Model file for the job. Use its own axes, mm. Face numbers are marked on the shaded views. A direction names the side the tool comes from. Give positions to 0.01 mm unless a question says otherwise; leave off trailing zeros. Order: outer loops, then holes, each group sorted by start corner. A loop starts at its lowest first (then second) coordinate and runs counter-clockwise, first axis right, second up. Notation, with made-up numbers: (66, 19.5) - (123, 19.5) arc R10 ccw to (123, 31.5) - close; hole circle Ø9 at (56.25, 34.5). An arc over 180 degrees is marked (long way). Use CSV: the item, a comma, the result in double quotes. Start each with the question number.
(1) Band-saw the part on C-C, the plane y = 5.5. Give the cut face in (x, z).
(2) Drop flat-ended pins along their axis: pin 1 Ø6 at (x, z) = (-13.5, 13.5) entering from +Y; pin 2 Ø1.7 at (y, z) = (-0.5, 119) entering from +X; pin 3 Ø6 at (x, z) = (58.5, 65) entering from -Y. Give the stop position or say it passes through.
(3) Band-saw the part on B-B, the plane x = -6.5. Give the cut face in (y, z).
(4) Tool access for the marked faces 5, 6 and 7: list every direction of +Z, -Z, +X, -X, +Y, -Y with a clear straight run to the whole face (end or side of a thin tool).
(5) Band-saw the part on A-A, the plane z = 12. Give the cut face in (x, y).
(6) Band-saw the part on D-D, the plane x = -44. Give the cut face in (y, z).
(7) Pull direction Z, two halves, no side cores. Call the marked faces 1, 2, 3 and 4: +Z half, -Z half, draft (parallel to the pull), parting line (faces both ways), or undercut.
(8) Probe L1, parallel to Z at x = 18.5, y = 8; L2, parallel to X at y = -4.5, z = 7.5; L3, parallel to Y at x = 47, z = 76.5. List the from-to ranges inside material, lowest first.
from build123d import *

# Parameters (mm, degrees)
F0_W         = 153.0012339354
F0_H         = 58.951575309
F1_DEPTH     = 20.32
F2_R         = 29.4340917525
F3_R         = 29.3662882484
F3_R_2       = 9.1215869303
F4_DEPTH     = 84.582
F5_DEPTH     = 84.583
F6_R         = 12.0800155098
F7_DEPTH     = 84.583
F9_W         = 152.801066637
F9_H         = 59.5563165843
F10_DEPTH    = 19.812
F11_R        = 10.3122867818
F12_DEPTH    = 124.461
F13_T1_DEPTH = 173.1145612107
F14_R        = 26.9812507731
F15_R        = 9.5592417263
F16_DEPTH    = 124.461


# Not quite as in the source:
# - a fillet or chamfer that OpenCascade refuses, or shapes differently, is made with other operations: its cross-section is extruded or revolved along the edge and cut away or added


with BuildPart() as f1:
    # F0 (on Top) → F1 (new body)
    with BuildSketch(Plane.XY):
        Rectangle(F0_W, F0_H)
    extrude(amount=F1_DEPTH)

    # F2
    f2_edges = [f1.edges().sort_by_distance(p)[0] for p in [
        (-76.500617, -29.475788, 10.16),
        (-76.500617, 29.475788, 10.16),
        (76.500617, -29.475788, 10.16),
        (76.500617, 29.475788, 10.16),
    ]]
    fillet(f2_edges, radius=F2_R)

    # F3 (on face) → F4 (join)
    with BuildSketch(Plane.XY.offset(20.32)):
        with Locations((47.0665252152, 0.0416959021)):
            Circle(F3_R)
        with Locations((47.0665252152, 0.0416959021)):
            Circle(F3_R_2, mode=Mode.SUBTRACT)
    extrude(amount=F4_DEPTH)

    # F5 (cut, through all): a face of the model
    f5_faces = [f1.faces().sort_by_distance(p)[0] for p in [
        (47.0665252152, 0.0416959021, 20.32),
    ]]
    extrude(f5_faces, amount=F5_DEPTH, mode=Mode.SUBTRACT)

    # F6 (on face) → F7 (cut, through all)
    with BuildSketch(Plane.XY.offset(20.32)):
        with Locations((-47.0665252152, 0.0416959021)):
            Circle(F6_R)
    extrude(amount=F7_DEPTH, mode=Mode.SUBTRACT)

    # F9 (on offset) → F10 (join)
    with BuildSketch(Plane.XY.offset(104.648)):
        Rectangle(F9_W, F9_H)
    extrude(amount=F10_DEPTH)

    # F11 (on face) → F12 (cut, through all)
    with BuildSketch(Plane(origin=(0, 0, 0), x_dir=(1, 0, 0), z_dir=(0, 0, -1))):
        with Locations((-47.0665252152, 0.0416959021)):
            Circle(F11_R)
    extrude(amount=-F12_DEPTH, mode=Mode.SUBTRACT)

    # F13: fillet of radius 30.6605122421 on 2 edges, made by hand

    # F13_s2 → F13_t1 (cut)
    with BuildSketch(Plane.XY.offset(27.9967193947)):
        with BuildLine():
            ThreePointArc((-45.7400210764, -29.7781582922), (-67.4202771975, -20.7979021711), (-76.4005333185, 0.88235395))
            Line((-76.4005333185, 0.88235395), (-76.4005333185, -29.7781582922))
            Line((-76.4005333185, -29.7781582922), (-45.7400210764, -29.7781582922))
        make_face()
        with BuildLine():
            ThreePointArc((-45.7400210764, 29.7781582922), (-67.4202771975, 20.7979021711), (-76.4005333185, -0.88235395))
            Line((-76.4005333185, -0.88235395), (-76.4005333185, 29.7781582922))
            Line((-76.4005333185, 29.7781582922), (-45.7400210764, 29.7781582922))
        make_face()
    extrude(amount=F13_T1_DEPTH, mode=Mode.SUBTRACT)

    # F14
    f14_edges = [f1.edges().sort_by_distance(p)[0] for p in [
        (76.400533, -29.778158, 114.554),
        (76.400533, 29.778158, 114.554),
    ]]
    fillet(f14_edges, radius=F14_R)

    # F15 (on face) → F16 (cut, through all)
    with BuildSketch(Plane(origin=(0, 0, 0), x_dir=(1, 0, 0), z_dir=(0, 0, -1))):
        with Locations((56.2476292253, 0)):
            Circle(F15_R)
    extrude(amount=-F16_DEPTH, mode=Mode.SUBTRACT)


solid = f1.part
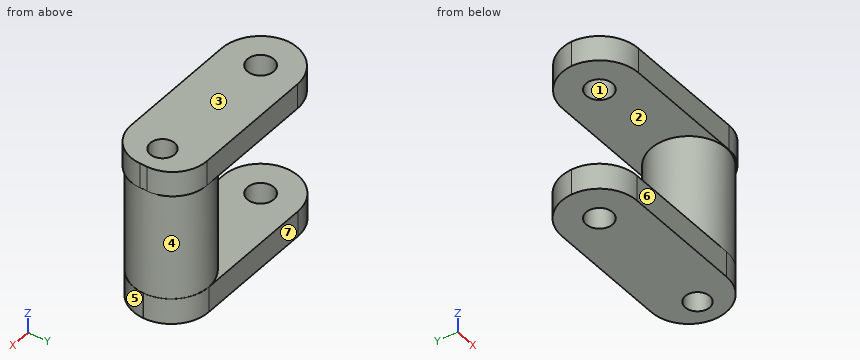
Answer block:
1,outline,"(-75.99, 0) - (-55.76, 0) - (-55.76, 20.32) - (-75.99, 20.32) - close; (-75.73, 104.65) - (-55.76, 104.65) - (-55.76, 124.46) - (-75.73, 124.46) - close; (-38.37, 0) - (48.43, 0) - (48.43, 20.32) - (39.76, 20.32) - (39.76, 104.65) - (48.43, 104.65) - (48.43, 124.46) - (-38.37, 124.46) - (-38.37, 104.65) - (18.21, 104.65) - (18.21, 20.32) - (-38.37, 20.32) - close; (64.07, 0) - (75.99, 0) - (75.99, 20.32) - (75.92, 20.32) - (75.92, 104.65) - (76.26, 104.65) - (76.26, 124.46) - (64.07, 124.46) - close"
2,pin 1,"stops at y = 29.48"
2,pin 2,"stops at x = 76.4"
2,pin 3,"stops at y = -28.09"
3,outline,"(-29.78, 104.65) - (29.78, 104.65) - (29.78, 124.46) - (-29.78, 124.46) - close; (-29.48, 0) - (29.48, 0) - (29.48, 20.32) - (-29.48, 20.32) - close"
4,face 5,"-Z, +X, -Y"
4,face 6,"-Z, +X, -X, -Y"
4,face 7,"-Z, +X, -X, +Y"
5,outline,"(-76.5, -0.04) arc R29.43 ccw to (-47.07, -29.48) - (47.07, -29.48) arc R29.43 ccw to (76.5, -0.04) - (76.5, 0.04) arc R29.43 ccw to (47.07, 29.48) - (-47.07, 29.48) arc R29.43 ccw to (-76.5, 0.04) - close; hole circle Ø20.62 at (-47.07, -0.04); hole circle Ø19.12 at (56.25, 0)"
6,outline,"(-29.78, 104.65) - (-9.89, 104.65) - (-9.89, 124.46) - (-29.78, 124.46) - close; (-29.48, 0) - (-9.89, 0) - (-9.89, 20.32) - (-29.48, 20.32) - close; (9.8, 0) - (29.48, 0) - (29.48, 20.32) - (9.8, 20.32) - close; (9.8, 104.65) - (29.78, 104.65) - (29.78, 124.46) - (9.8, 124.46) - close"
7,face 1,"draft"
7,face 2,"undercut"
7,face 3,"+Z half"
7,face 4,"undercut"
8,L1,"z = 0 to 20.32, 104.65 to 124.46"
8,L2,"x = -76.16 to -56.37, -37.77 to 47.81, 64.68 to 76.16"
8,L3,"y = -29.32 to -9.08, 9.16 to 29.41"
